```python
from build123d import *

# Parameters (mm, degrees)
SKETCH1_W                   = 140
SKETCH1_H                   = 120
LID_EXTRUDE_DEPTH           = 10
SKETCH3_W                   = 5
SKETCH3_H                   = 95
LOCATION_BAR_EXTRUDE_DEPTH  = 10
M6_TAPPED_HOLE1_D           = 5
M6_TAPPED_HOLE1_CSINK_D     = 6.05
M6_TAPPED_HOLE1_CSINK_ANGLE = 90
MOTOR_HOLE_CUT_REACH        = 96.34
SKETCH6_R                   = 16
FILLET2_R                   = 1


with BuildPart() as part:
    # Sketch1 → LID_EXTRUDE (new body)
    with BuildSketch(Plane(origin=(0, 0, 0), x_dir=(1, 0, 0), z_dir=(0, 1, 0))):
        Rectangle(SKETCH1_W, SKETCH1_H)
    extrude(amount=LID_EXTRUDE_DEPTH)

    # Sketch3 → LOCATION_BAR_EXTRUDE (add)
    with BuildSketch(Plane(origin=(0, 10, 0), x_dir=(1, 0, 0), z_dir=(0, 1, 0))):
        with Locations((-55.5, 0)):
            Rectangle(SKETCH3_W, SKETCH3_H)
        with Locations((55.5, 0)):
            Rectangle(SKETCH3_W, SKETCH3_H)
    extrude(amount=LOCATION_BAR_EXTRUDE_DEPTH)

    # M6 Tapped Hole1 (through all)
    with Locations(Plane(origin=(0, 0, 55), x_dir=(0, 0, -1), z_dir=(0, -1, 0))):
        with Locations((0, 0), (55, -65)):
            m6_tapped_hole1 = CounterSinkHole(M6_TAPPED_HOLE1_D / 2, M6_TAPPED_HOLE1_CSINK_D / 2, counter_sink_angle=M6_TAPPED_HOLE1_CSINK_ANGLE)

    # Mirror1: M6 Tapped Hole1 across plane
    add(m6_tapped_hole1.mirror(Plane(origin=(0, 0, 0), x_dir=(0, 0, 1), z_dir=(1, 0, 0))), mode=Mode.SUBTRACT)

    # Mirror1 at the second plane: M6 Tapped Hole1 across plane
    add(m6_tapped_hole1.mirror(Plane.XY), mode=Mode.SUBTRACT)

    # Sketch6 → MOTOR_HOLE_CUT (cut, up to next)
    with BuildSketch(Plane.XZ, mode=Mode.PRIVATE) as motor_hole_cut_sk1:
        with Locations(Location((15, 0, 0), (0, 0, 270))):
            Circle(SKETCH6_R)
    motor_hole_cut_tool1 = extrude(motor_hole_cut_sk1.sketch, amount=-MOTOR_HOLE_CUT_REACH, mode=Mode.PRIVATE) & part.part
    add(motor_hole_cut_tool1.solids().sort_by_distance((15, 0, 0))[0], mode=Mode.SUBTRACT)

    # Fillet2
    fillet2_edges = [part.edges().sort_by_distance(p)[0] for p in [
        (70, 10, 0),
        (0, 10, -60),
        (-70, 10, 0),
        (0, 0, -60),
        (70, 0, 0),
        (0, 0, 60),
        (-70, 0, 0),
        (0, 10, 60),
    ]]
    fillet(fillet2_edges, radius=FILLET2_R)


solid = part.part
```
Could you check a few things on this model? Use its own coordinates, in mm. A direction names the side the tool comes from. Give positions to 0.01 mm unless a question says otherwise; leave off trailing zeros. Write each loop counter-clockwise with the first axis right and the second up, starting at its lowest first coordinate (ties: lowest second). Pieces come first, ordered by that corner, then holes. Notation, with made-up numbers: (38, -13) - (95, -13) arc R6 cw to (95, -4) - close; hole circle Ø2 at (55, 78.5). An arc over 180 degrees is marked (long way). One line per item, written item: value. Start each with the question number.
Item 1: Imagine slicing it at C-C, the plane y = 3. List the corners of the cut face in (x, z) for me.
Item 2: Which directions (+Z, -Z, +X, -X, +Y, -Y) give clear straight access to the entire face, cutting with the end or side of a thin tool? Please do faces 5 (the face through (-70, 5, 1)), 6 (the face through (55, 15, -47.5)), 7 (the face through (-53, 15, 1)).
Item 3: Please list where these lines run through material, in increasing order: line 1 (X direction, y = 2.75, z = 0); line 2 (X direction, y = 19.25, z = -45.5); line 3 (X direction, y = 8.25, z = 55). Write a range as from..to.
Item 4: Imagine slicing it at D-D, the plane z = -55. List the corners of the cut face in (x, y) for me (3 decimals).
Item 5: If we mould it in two halves opening along Z, with no side actions, what happens to faces 1 (the face through (-58, 15, 1)), 2 (the face through (-67.22, 5.33, 1.15)), 3 (the face through (55, 15, 47.5)), 4 (the face through (63.31, 5.33, -1.84))? For each: +Z half, -Z half, draft (parallel to the pull), parting line (faces both ways), or undercut.
Item 6: Imagine slicing it at B-B, the plane z = 0. Give the number of separate pieces and of enclosed holes in the cut face, and give its area (3 significant figures).
Item 7: Imagine slicing it at A-A, the plane x = 15. List the corners of the cut face in (y, z) for me, and give its area (3 significant figures).
Item 8: I'm going to push flat-ended pins straight in: pin 1 (6.5 mm diameter, centred on x = 0, z = 55, fed in from +Y); pin 2 (4 mm diameter, centred on x = 56, y = 15.5, fed in from +Z); pin 3 (11 mm diameter, centred on y = 15, z = -16.5, fed in from -X). Where does each tip first touch, or does it pass through?
Geometry says:
1. outline: (-70, -60) - (70, -60) - (70, 60) - (-70, 60) - close; hole circle Ø5 at (-65, 0); hole circle Ø5 at (0, -55); hole circle Ø5 at (0, 55); hole circle Ø32 at (15, 0); hole circle Ø5 at (65, 0)
2. face 5: +Z, -Z, -X, +Y, -Y
2. face 6: -Z, +X, -X, +Y
2. face 7: +Z, -Z, +Y
3. line 1: -70..-67.5, -62.5..-1, 31..62.5, 67.5..70
3. line 2: -58..-53, 53..58
3. line 3: -70..-2.5, 2.5..70
4. outline: (-70, 1) arc R1 ccw to (-69, 0) - (-3.025, 0) - (-2.5, 0.525) - (-2.5, 10) - (-69, 10) arc R1 ccw to (-70, 9) - close; (2.5, 0.525) - (3.025, 0) - (69, 0) arc R1 ccw to (70, 1) - (70, 9) arc R1 ccw to (69, 10) - (2.5, 10) - close
5. face 1: draft
5. face 2: undercut
5. face 3: +Z half
5. face 4: undercut
6. separate pieces: 4
6. enclosed holes: 0
6. area: 1,080 mm^2
7. outline: (0, -59) arc R1 ccw to (1, -60) - (9, -60) arc R1 ccw to (10, -59) - (10, -16) - (0, -16) - close; (0, 16) - (10, 16) - (10, 59) arc R1 ccw to (9, 60) - (1, 60) arc R1 ccw to (0, 59) - close
7. area: 879 mm^2
8. pin 1: y = 10
8. pin 2: z = 47.5
8. pin 3: x = -69.87
